```python
from build123d import *

# Parameters (mm, degrees)
SKETCH1_W            = 60
SKETCH1_H            = 42
BOSS_EXTRUDE1_DEPTH  = 8
SKETCH3_W            = 10
SKETCH3_H            = 42
BOSS_EXTRUDE5_DEPTH  = 6
SKETCH5_W            = 14
SKETCH5_H            = 42
BOSS_EXTRUDE6_DEPTH  = 11
SKETCH6_R            = 3.2
CUT_EXTRUDE1_DEPTH   = 75.565407529
FILLET1_R            = 7
FILLET2_R            = 5
FILLET3_R            = 5
BOSS_EXTRUDE7_DEPTH  = 42
SKETCH9_W            = 5
SKETCH9_H            = 42
BOSS_EXTRUDE8_DEPTH  = 6
SKETCH11_W           = 15
SKETCH11_H           = 42
CUT_EXTRUDE2_DEPTH   = 76.921011584
SKETCH12_W           = 30
SKETCH12_H           = 42
CUT_EXTRUDE3_DEPTH   = 6
SKETCH15_W           = 42
SKETCH15_H           = 8
BOSS_EXTRUDE9_DEPTH  = 5
SKETCH16_W           = 42
SKETCH16_H           = 8
BOSS_EXTRUDE10_DEPTH = 5
CUT_EXTRUDE7_START   = -17
CUT_EXTRUDE7_DEPTH   = 17
BOSS_EXTRUDE11_START = -5
SKETCH17_R           = 4.15
SKETCH17_R_2         = 2.2
BOSS_EXTRUDE11_DEPTH = 5
SKETCH18_W           = 2
SKETCH18_H           = 42
CUT_EXTRUDE8_DEPTH   = 67.392770772
CUT_EXTRUDE9_DEPTH   = 3
CUT_EXTRUDE10_START  = -3
CUT_EXTRUDE10_DEPTH  = 3


with BuildPart() as part:
    # Sketch1 → Boss-Extrude1 (new body)
    with BuildSketch(Plane(origin=(0, 0, 0), x_dir=(1, 0, 0), z_dir=(0, 1, 0))):
        with Locations((30, 21)):
            Rectangle(SKETCH1_W, SKETCH1_H)
    extrude(amount=BOSS_EXTRUDE1_DEPTH)

    # Sketch3 → Boss-Extrude5 (add)
    with BuildSketch(Plane(origin=(0, 8, 0), x_dir=(1, 0, 0), z_dir=(0, 1, 0))):
        with Locations((30, 21)):
            Rectangle(SKETCH3_W, SKETCH3_H)
    extrude(amount=BOSS_EXTRUDE5_DEPTH)

    # Sketch5 → Boss-Extrude6 (add)
    with BuildSketch(Plane.XZ):
        with Locations((30, -21)):
            Rectangle(SKETCH5_W, SKETCH5_H)
    extrude(amount=BOSS_EXTRUDE6_DEPTH)

    # Sketch6 → Cut-Extrude1 (cut, through all)
    with BuildSketch(Plane(origin=(0, 0, -42), x_dir=(-1, 0, 0), z_dir=(0, 0, -1))):
        with Locations((-30, -5)):
            Circle(SKETCH6_R)
    extrude(amount=-CUT_EXTRUDE1_DEPTH, mode=Mode.SUBTRACT)

    # Fillet1
    fillet1_edges = [part.edges().sort_by_distance(p)[0] for p in [
        (23, -11, -21),
        (37, -11, -21),
    ]]
    fillet(fillet1_edges, radius=FILLET1_R - 0.0001)  # a hair under: the kernel refuses the full size

    # Fillet2
    fillet2_edges = [part.edges().sort_by_distance(p)[0] for p in [
        (23, 0, -21),
    ]]
    fillet(fillet2_edges, radius=FILLET2_R)

    # Fillet3
    fillet3_edges = [part.edges().sort_by_distance(p)[0] for p in [
        (37, 0, -21),
    ]]
    fillet(fillet3_edges, radius=FILLET3_R)

    # Sketch8 → Boss-Extrude7 (add)
    with BuildSketch(Plane(origin=(0, 0, -42), x_dir=(-1, 0, 0), z_dir=(0, 0, -1))):
        with BuildLine():
            Line((-41.958260743, -1), (-42.958260743, 0))
            Line((-42.958260743, 0), (-41.958260743, 0))
            ThreePointArc((-41.958260743, 0), (-38.573244741, -1.320099639), (-36.9756521, -4.583333333))
            ThreePointArc((-36.9756521, -4.583333333), (-34.739022403, -9.151860505), (-30, -11))
            ThreePointArc((-30, -11), (-25.260977597, -9.151860505), (-23.0243479, -4.583333333))
            ThreePointArc((-23.0243479, -4.583333333), (-21.426755259, -1.320099639), (-18.041739257, 0))
            Line((-18.041739257, 0), (-16.803044796, 0))
            Line((-16.803044796, 0), (-18.041739257, -1))
            ThreePointArc((-18.041739257, -1), (-20.749752058, -2.056079711), (-22.027826171, -4.666666667))
            ThreePointArc((-22.027826171, -4.666666667), (-24.583974397, -9.887840578), (-30, -12))
            ThreePointArc((-30, -12), (-35.416025603, -9.887840578), (-37.972173829, -4.666666667))
            ThreePointArc((-37.972173829, -4.666666667), (-39.250247942, -2.056079711), (-41.958260743, -1))
        make_face()
    extrude(amount=-BOSS_EXTRUDE7_DEPTH)

    # Sketch9 → Boss-Extrude8 (add)
    with BuildSketch(Plane(origin=(0, 8, 0), x_dir=(1, 0, 0), z_dir=(0, 1, 0))):
        with Locations((42.5, 21)):
            Rectangle(SKETCH9_W, SKETCH9_H)
        with Locations((17.5, 21)):
            Rectangle(SKETCH9_W, SKETCH9_H)
    extrude(amount=BOSS_EXTRUDE8_DEPTH)

    # Sketch11 → Cut-Extrude2 (cut, through all)
    with BuildSketch(Plane(origin=(0, 8, 0), x_dir=(1, 0, 0), z_dir=(0, 1, 0))):
        with Locations((52.5, 21)):
            Rectangle(SKETCH11_W, SKETCH11_H)
        with Locations((7.5, 21)):
            Rectangle(SKETCH11_W, SKETCH11_H)
    extrude(amount=-CUT_EXTRUDE2_DEPTH, mode=Mode.SUBTRACT)

    # Sketch12 → Cut-Extrude3 (cut)
    with BuildSketch(Plane(origin=(0, 14, 0), x_dir=(1, 0, 0), z_dir=(0, 1, 0))):
        with Locations((30, 21)):
            Rectangle(SKETCH12_W, SKETCH12_H)
    extrude(amount=-CUT_EXTRUDE3_DEPTH, mode=Mode.SUBTRACT)

    # Sketch15 → Boss-Extrude9 (add)
    with BuildSketch(Plane.ZY.offset(-15)):
        with Locations((-21, 4)):
            Rectangle(SKETCH15_W, SKETCH15_H)
    extrude(amount=BOSS_EXTRUDE9_DEPTH)

    # Sketch16 → Boss-Extrude10 (add)
    with BuildSketch(Plane(origin=(45, 0, 0), x_dir=(0, 0, -1), z_dir=(1, 0, 0))):
        with Locations((21, 4)):
            Rectangle(SKETCH16_W, SKETCH16_H)
    extrude(amount=BOSS_EXTRUDE10_DEPTH)

    # Cut-Extrude7: read off the stored shape, not the designer's step
    # Cut-Extrude7 outline → Cut-Extrude7 (cut)
    with BuildSketch(Plane(origin=(0, 8, 0), x_dir=(1, 0, 0), z_dir=(0, 1, 0)).offset(CUT_EXTRUDE7_START)):
        with BuildLine():
            ThreePointArc((45, 33.105667219), (36.85, 32), (45, 30.894332781))
            Line((45, 30.894332781), (45, 33.105667219))
        make_face()
        with BuildLine():
            ThreePointArc((45, 11.105667219), (36.85, 10), (45, 8.894332781))
            Line((45, 8.894332781), (45, 11.105667219))
        make_face()
        with BuildLine():
            ThreePointArc((15, 8.894332781), (23.15, 10), (15, 11.105667219))
            Line((15, 11.105667219), (15, 8.894332781))
        make_face()
        with BuildLine():
            ThreePointArc((15, 30.894332781), (23.15, 32), (15, 33.105667219))
            Line((15, 33.105667219), (15, 30.894332781))
        make_face()
    extrude(amount=CUT_EXTRUDE7_DEPTH, mode=Mode.SUBTRACT)

    # Sketch17 → Boss-Extrude11 (add)
    # profile 1 of 4: a face of its own
    with BuildSketch(Plane(origin=(0, 8, 0), x_dir=(1, 0, 0), z_dir=(0, 1, 0)).offset(BOSS_EXTRUDE11_START)):
        with Locations((41, 32)):
            Circle(SKETCH17_R)
        with Locations(Location((41, 32, 0), (0, 0, 270))):
            Circle(SKETCH17_R_2, mode=Mode.SUBTRACT)
    # profile 2 of 4: a face of its own
    with BuildSketch(Plane(origin=(0, 8, 0), x_dir=(1, 0, 0), z_dir=(0, 1, 0)).offset(BOSS_EXTRUDE11_START)):
        with Locations((19, 10)):
            Circle(SKETCH17_R)
        with Locations(Location((19, 10, 0), (0, 0, 270))):
            Circle(SKETCH17_R_2, mode=Mode.SUBTRACT)
    # profile 3 of 4: a face of its own
    with BuildSketch(Plane(origin=(0, 8, 0), x_dir=(1, 0, 0), z_dir=(0, 1, 0)).offset(BOSS_EXTRUDE11_START)):
        with Locations((41, 10)):
            Circle(SKETCH17_R)
        with Locations(Location((41, 10, 0), (0, 0, 270))):
            Circle(SKETCH17_R_2, mode=Mode.SUBTRACT)
    # profile 4 of 4: a face of its own
    with BuildSketch(Plane(origin=(0, 8, 0), x_dir=(1, 0, 0), z_dir=(0, 1, 0)).offset(BOSS_EXTRUDE11_START)):
        with Locations((19, 32)):
            Circle(SKETCH17_R)
        with Locations(Location((19, 32, 0), (0, 0, 270))):
            Circle(SKETCH17_R_2, mode=Mode.SUBTRACT)
    extrude(amount=BOSS_EXTRUDE11_DEPTH)

    # Sketch18 → Cut-Extrude8 (cut, through all)
    with BuildSketch(Plane.XZ):
        with Locations((11, -21)):
            Rectangle(SKETCH18_W, SKETCH18_H)
        with Locations((49, -21)):
            Rectangle(SKETCH18_W, SKETCH18_H)
    extrude(amount=-CUT_EXTRUDE8_DEPTH, mode=Mode.SUBTRACT)

    # Sketch20 → Cut-Extrude9 (cut)
    with BuildSketch(Plane(origin=(0, 0, -42), x_dir=(-1, 0, 0), z_dir=(0, 0, -1))):
        with BuildLine():
            Line((-16.803044796, 0), (-12, 0))
            Line((-12, 0), (-12, 8))
            Line((-12, 8), (-48, 8))
            Line((-48, 8), (-48, 0))
            Line((-48, 0), (-42.958260743, 0))
            Line((-42.958260743, 0), (-41.958260743, -1))
            ThreePointArc((-41.958260743, -1), (-39.250247942, -2.056079711), (-37.972173829, -4.666666667))
            ThreePointArc((-37.972173829, -4.666666667), (-30, -12), (-22.027826171, -4.666666667))
            ThreePointArc((-22.027826171, -4.666666667), (-20.749752058, -2.056079711), (-18.041739257, -1))
            Line((-18.041739257, -1), (-16.803044796, 0))
        make_face()
    extrude(amount=-CUT_EXTRUDE9_DEPTH, mode=Mode.SUBTRACT)

    # Sketch19 → Cut-Extrude10 (cut)
    with BuildSketch(Plane.XY.offset(CUT_EXTRUDE10_START)):
        with BuildLine():
            Line((48, 8), (12, 8))
            Line((12, 8), (12, 0))
            Line((12, 0), (16.803044796, 0))
            Line((16.803044796, 0), (18.041739257, -1))
            ThreePointArc((18.041739257, -1), (20.749752058, -2.056079711), (22.027826171, -4.666666667))
            ThreePointArc((22.027826171, -4.666666667), (30, -12), (37.972173829, -4.666666667))
            ThreePointArc((37.972173829, -4.666666667), (39.250247942, -2.056079711), (41.958260743, -1))
            Line((41.958260743, -1), (42.958260743, 0))
            Line((42.958260743, 0), (48, 0))
            Line((48, 0), (48, 8))
        make_face()
    extrude(amount=CUT_EXTRUDE10_DEPTH, mode=Mode.SUBTRACT)


solid = part.part
```
For this review, take the finished solid that the model builds, in its own axes (mm). A direction names the side the tool comes from. Round coordinates to 2 decimals unless told otherwise and drop trailing zeros. Write each loop counter-clockwise with the first axis right and the second up, starting at its lowest first coordinate (ties: lowest second). Pieces come first, ordered by that corner, then holes.
1) Take a section at D-D on x = 19. Give the boundary of the cut face in (y, z).
Answer below:
outline: (-1.12, -39) - (8, -39) - (8, -34.2) - (3, -34.2) - (3, -36.15) - (-1.12, -36.15) - close; (-1.12, -27.85) - (3, -27.85) - (3, -29.8) - (8, -29.8) - (8, -12.2) - (3, -12.2) - (3, -14.15) - (-1.12, -14.15) - close; (-1.12, -5.85) - (3, -5.85) - (3, -7.8) - (8, -7.8) - (8, -3) - (-1.12, -3) - close
2) Insertion check: pin 1 Ø12 at (y, z) = (-3.5, -24.5) entering from +X; pin 2 Ø5.5 at (x, z) = (14, -12.5) entering from -Y; pin 3 Ø5.5 at (x, z) = (19, -10) entering from -Y; pin 4 Ø2.5 at (x, z) = (41, -32) entering from +Y. Each pin has a flat end and moves straight along its axis. Give the tip position at first contact, or say it passes through.
Answer below:
pin 1: stops at x = 48
pin 2: stops at y = 0
pin 3: stops at y = 3
pin 4: passes through
3) Take a section at B-B on y = 3.5. Give the boundary of the cut face in (x, z).
Answer below:
outline: (12, -39) - (48, -39) - (48, -3) - (12, -3) - close; hole circle Ø4.4 at (19, -32); hole circle Ø4.4 at (19, -10); hole circle Ø4.4 at (41, -32); hole circle Ø4.4 at (41, -10)
4) For line 1 along X through (y, z) = (5.25, -32); line 2 along Z through (x, y) = (22, 2); line 3 along X through (y, z) = (7.25, -9.5), list the stretches that pass through material, from the lowest coordinate up.
Answer below:
line 1: x = 12 to 16.8, 21.2 to 38.8, 43.2 to 48
line 2: z = -39 to -34.87, -29.13 to -12.87, -7.13 to -3
line 3: x = 12 to 16.86, 21.14 to 38.86, 43.14 to 48
5) Mouldability with a two-part tool opening along X and no side actions: class faces 4 (the face through (17.41, -0.49, -37.28)), 5 (the face through (39.22, -2.084, -37.411)), 6 (the face through (33.2, -4.9, -21.3)), 7 (the face through (36.853, -0.17, -10.167)) as +X half, -X half, draft (parallel to the pull), parting line (faces both ways), or undercut.
Answer below:
face 4: -X half
face 5: +X half
face 6: undercut
face 7: undercut
6) Take a section at C-C on z = -22. Give the boundary of the cut face in (x, y), then the cut area to 3 significant figures.
Answer below:
outline: (12, 0) - (16.8, 0) - (18.04, -1) arc R4 cw to (22.03, -4.67) arc R8 ccw to (37.97, -4.67) arc R4 cw to (41.96, -1) - (42.96, 0) - (48, 0) - (48, 8) - (12, 8) - close; hole circle Ø6.4 at (30, -5)
area: 436 mm2
7) Take a section at A-A on z = -10. Give the boundary of the cut face in (x, y).
Answer below:
outline: (12, 0) - (15, 0) - (15, 3) - (16.8, 3) - (16.8, 8) - (12, 8) - close; (21.2, 3) - (23.15, 3) - (23.15, -8.13) arc R8 ccw to (36.85, -8.13) - (36.85, 3) - (38.8, 3) - (38.8, 8) - (21.2, 8) - close; (43.2, 3) - (45, 3) - (45, 0) - (48, 0) - (48, 8) - (43.2, 8) - close; hole circle Ø6.4 at (30, -5)
8) Machinability: for faces 1 (the face through (23.147, -1.407, -9.833)), 2 (the face through (20.72, -2.03, -21.11)), 3 (the face through (45, 0, -21)), which of the approach directions +Z, -Z, +X, -X, +Y, -Y give a long, thin tool a straight path to every point of the face, cutting with its end or side? Answer none if there is none.
Answer below:
face 1: -Y
face 2: +Z, -Z, -X, -Y
face 3: +Z, -Z, +X, -Y
